Read the model definition and answer for the solid it produces. Units are mm, in the model's axes. A direction names the side the tool comes from. Give positions to 0.01 mm unless a question says otherwise; leave off trailing zeros. Order: outer loops, then holes, each group sorted by start corner. A loop starts at its lowest first (then second) coordinate and runs counter-clockwise, first axis right, second up. Notation, with made-up numbers: (-16, -11) - (17, -11) arc R16 ccw to (17, -5) - close; hole circle Ø5 at (5, 20). An arc over 180 degrees is marked (long way). Write each question's results on one line, items separated by ' | '. Start each with the question number.
Q1. Find section D-D on x = -11. Give the vertices of the cut face in (y, z), and give its area (3 significant figures).
Q2. For a pull along X with two mould halves and no side action, classify faces 5 (the face through (-15, -4, 0)), 6 (the face through (-19.499, 2.922, 14.177)), 7 (the face through (-12.277, -21.208, 9.86)) as +X half, -X half, draft (parallel to the pull), parting line (faces both ways), or undercut.
Q3. Find section B-B on z = 5. Count the separate pieces of the cut face and the enclosed holes in it, and give its area (3 significant figures).
Q4. Find section C-C on y = -8.5. Give the vertices of the cut face in (x, z).
Q5. Find section A-A on x = 0. Give the vertices of the cut face in (y, z), and give its area (3 significant figures).
Q6. Find the intervals of material crossed by line 1 along Y through (x, z) = (0, 5.75); line 2 along Y through (x, z) = (-4, 5); line 3 along X through (y, z) = (6.5, 4.5), in increasing order. Write a range as from..to.
Q7. Flat-ended cylindrical pins translate along their axes: P1, Ø5, axis at x = -21.48, z = 5, coming from the -Y side; P2, Ø6, axis at y = 15.5, z = 3, coming from the -X side; P3, Ø3, axis at x = 0, y = -14.5, coming from the -Z side; P4, Ø10, axis at x = -19, z = 14.5, coming from the -Y side. Find the tip coordinate at first contact, or state that the pin passes through.
Q8. A tool of negligible diameter and unlimited length cuts with its end or side. For faces 1 (the face through (-12.21, -17.15, 5.7)), 2 (the face through (-8.749, 19.153, 5.696)), 3 (the face through (21, -2, 6)), 4 (the face through (21, 2, 6)), from which of +Z, -Z, +X, -X, +Y, -Y can it reach the whole face along a straight path? Write none if from no direction.
from build123d import *

# Parameters (mm, degrees)
PAD_DEPTH          = 20
SKETCH001_R        = 2.15
POCKET_DEPTH       = 17.001
POCKET_DEPTH_BACK  = -17.001
PAD001_DEPTH       = 2
POLARPATTERN_COUNT = 3
POLARPATTERN_ANGLE = 240


with BuildPart() as part:
    # Sketch → Pad (new body)
    with BuildSketch(Plane.XY):
        with BuildLine():
            ThreePointArc((-14.96663, -1), (15, 0), (-14.96663, 1))
            Line((-14.96663, 1), (-26.673727, 1.782213))
            Line((-26.673727, 1.782213), (-26.473727, 4.775539))
            Line((-26.473727, 4.775539), (-16.495974, 4.108873))
            ThreePointArc((-16.495974, -4.108873), (17, 0), (-16.495974, 4.108873))
            Line((-26.473727, -4.775539), (-16.495974, -4.108873))
            Line((-26.673727, -1.782213), (-26.473727, -4.775539))
            Line((-14.96663, -1), (-26.673727, -1.782213))
        make_face()
    extrude(amount=PAD_DEPTH)

    # Sketch001 → Pocket (cut, two sides)
    with BuildSketch(Plane.XZ) as pocket_sk:
        with Locations((-21.484851, 15)):
            Circle(SKETCH001_R)
        with Locations((-21.484851, 5)):
            Circle(SKETCH001_R)
    extrude(amount=-POCKET_DEPTH, mode=Mode.SUBTRACT)
    extrude(pocket_sk.sketch, amount=-POCKET_DEPTH_BACK, mode=Mode.SUBTRACT)

    # Sketch002 → Pad001 (join, symmetric)
    with BuildSketch(Plane.XZ):
        Polygon((16.9, 20), (16.9, 0), (31.9, 0), align=None)
    pad001 = extrude(amount=PAD001_DEPTH, both=True)

    # PolarPattern: Pad001 ×3 about axis
    polarpattern_axis = Axis((0, 0, 0), (0, 0, 1))
    for i in range(1, POLARPATTERN_COUNT):
        add(pad001.rotate(polarpattern_axis, i * POLARPATTERN_ANGLE / (POLARPATTERN_COUNT - 1)))


solid = part.part
Working result:
1) outline: (-23.05, 0) - (-15.05, 0) - (-15.05, 17.82) - (-23.05, 8.58) - close; (-12.96, 0) - (-10.2, 0) - (-10.2, 20) - (-12.96, 20) - close; (10.2, 0) - (12.96, 0) - (12.96, 20) - (10.2, 20) - close; (15.05, 0) - (23.05, 0) - (23.05, 8.58) - (15.05, 17.82) - close | area: 322 mm²
2) face 5: draft | face 6: undercut | face 7: -X half
3) separate pieces: 3 | enclosed holes: 0 | area: 364 mm²
4) outline: (-14.72, 0) - (-12.36, 0) - (-12.36, 20) - (-14.72, 20) - close; (12.36, 0) - (14.72, 0) - (14.72, 20) - (12.36, 20) - close
5) outline: (-17, 0) - (-15, 0) - (-15, 20) - (-17, 20) - close; (15, 0) - (17, 0) - (17, 20) - (15, 20) - close | area: 80.0 mm²
6) line 1: -17..-15, 15..17 | line 2: -16.52..-14.46, 14.46..16.52 | line 3: -15.71..-13.52, 13.52..15.71
7) P1: y = -4.61 | P2: x = -12.99 | P3: z = 0 | P4: y = -9.64
8) face 1: +Z, -Z, -X | face 2: +Z, -Z, +Y | face 3: +Z, -Z, +X, -Y | face 4: +Z, -Z, +X, +Y
